Check sheet for the modelled part. Datum: model origin and axes. Units: mm. Give positions to 0.01 mm unless a question says otherwise; leave off trailing zeros. Loops run counter-clockwise (first coordinate to the right, second up) from the corner with the lowest first, then second, coordinate; pieces in that order, holes last.
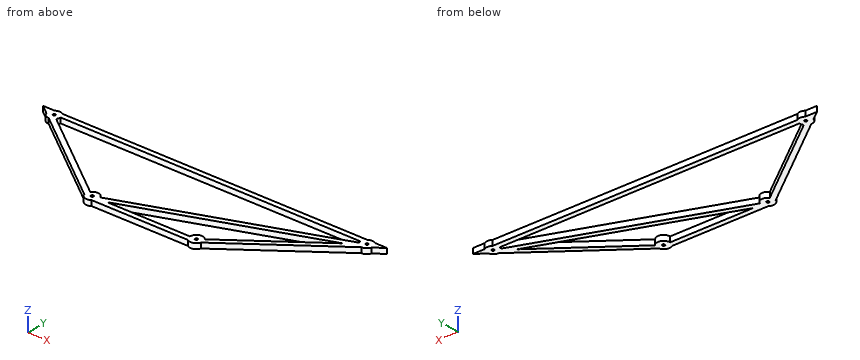
```python
from build123d import *

# Parameters (mm, degrees)
EXTRUDE_THIN2_DEPTH = 20
SKETCH4_R           = 5
CUT_EXTRUDE1_DEPTH  = 1302.393483924


# Read off the part's stored shape, not the designer's step: Extrude-Thin2
with BuildPart() as part:
    # Extrude-Thin2 outline → Extrude-Thin2 (new body)
    with BuildSketch(Plane.XY):
        with BuildLine():
            Line((-15, 20), (-60, 20))
            Line((-60, 20), (-24, -7))
            ThreePointArc((-24, -7), (-15, -20), (0, -25))
            Line((0, -25), (376, -307))
            ThreePointArc((376, -307), (392.09430585, -323.717082451), (415, -320))
            Line((415, -320), (785, -320))
            ThreePointArc((785, -320), (807.90569415, -323.717082451), (824, -307))
            Line((824, -307), (1200, -25))
            ThreePointArc((1200, -25), (1215, -20), (1224, -7))
            Line((1224, -7), (1260, 20))
            Line((1260, 20), (1215, 20))
            ThreePointArc((1215, 20), (1200, 25), (1185, 20))
            Line((1185, 20), (15, 20))
            ThreePointArc((15, 20), (0, 25), (-15, 20))
        make_face()
        with BuildLine():
            Line((456.960024969, -300), (1143.039975031, -42.720018727))
            Line((1143.039975031, -42.720018727), (820, -285))
            ThreePointArc((820, -285), (792.09430585, -276.282917549), (775, -300))
            Line((775, -300), (456.960024969, -300))
        make_face(mode=Mode.SUBTRACT)
        with BuildLine():
            ThreePointArc((1175, 0), (1175.401161247, -4.460620138), (1176.591770561, -8.77808604))
            Line((1176.591770561, -8.77808604), (423.408229439, -291.22191396))
            ThreePointArc((423.408229439, -291.22191396), (403.547120002, -275.252920583), (380, -285))
            Line((380, -285), (20, -15))
            ThreePointArc((20, -15), (23.717082451, -7.90569415), (25, 0))
            Line((25, 0), (1175, 0))
        make_face(mode=Mode.SUBTRACT)
    extrude(amount=EXTRUDE_THIN2_DEPTH)

    # Sketch4 → Cut-Extrude1 (cut, through all)
    with BuildSketch(Plane.XY.offset(20)):
        Circle(SKETCH4_R)
        with Locations((400, -300)):
            Circle(SKETCH4_R)
        with Locations((800, -300)):
            Circle(SKETCH4_R)
        with Locations((1200, 0)):
            Circle(SKETCH4_R)
    extrude(amount=-CUT_EXTRUDE1_DEPTH, mode=Mode.SUBTRACT)


solid = part.part
```
(1) Gauge pin test, flat ends, axial feed: pin 1 Ø2 at (x, z) = (144.5, 11) entering from +Y; pin 2 Ø6 at (x, z) = (515, 11.5) entering from -Y; pin 3 Ø12 at (y, z) = (-17, 12.5) entering from +X. Record the tip position at first contact, or that the pin passes through.
(2) Section check A-A on z = 13. Record the boundary of the cut face in (x, y), plus the area to 3 significant figures.
(3) Material ranges on line 1 (Y direction, x = 400, z = 8.25); line 2 (Y direction, x = 601.5, z = 5.25); line 3 (Y direction, x = 1200, z = 13), recorded low to high.
(4) Section check D-D on x = 654.5. Record the boundary of the cut face in (y, z).
(5) Section check C-C on y = -112.5. Record the boundary of the cut face in (x, z).
(6) Section check B-B on x = 89.5. Record the boundary of the cut face in (y, z) (3 decimals), plus the area to 3 significant figures.
Computed values:
1. pin 1: stops at y = 20
1. pin 2: stops at y = -320
1. pin 3: stops at x = 1222.45
2. outline: (-60, 20) - (-24, -7) arc R25 ccw to (0, -25) - (376, -307) arc R25 ccw to (415, -320) - (785, -320) arc R25 ccw to (824, -307) - (1200, -25) arc R25 ccw to (1224, -7) - (1260, 20) - (1215, 20) arc R25 ccw to (1185, 20) - (15, 20) arc R25 ccw to (-15, 20) - close; hole circle Ø10 at (0, 0); hole (20, -15) - (380, -285) arc R25 cw to (423.41, -291.22) - (1176.59, -8.78) arc R25 cw to (1175, 0) - (25, 0) arc R25 cw to start; hole circle Ø10 at (400, -300); hole (456.96, -300) - (775, -300) arc R25 cw to (820, -285) - (1143.04, -42.72) - close; hole circle Ø10 at (800, -300); hole circle Ø10 at (1200, 0)
2. area: 72,700 mm2
3. line 1: y = -325 to -305, -295 to -275, 0 to 20
3. line 2: y = -320 to -300, -245.8 to -224.44, 0 to 20
3. line 3: y = -25 to -5, 5 to 25
4. outline: (-320, 0) - (-300, 0) - (-300, 20) - (-320, 20) - close; (-225.92, 0) - (-204.56, 0) - (-204.56, 20) - (-225.92, 20) - close; (0, 0) - (20, 0) - (20, 20) - (0, 20) - close
5. outline: (116.67, 0) - (150, 0) - (150, 20) - (116.67, 20) - close; (900, 0) - (956.96, 0) - (956.96, 20) - (900, 20) - close; (1050, 0) - (1083.33, 0) - (1083.33, 20) - (1050, 20) - close
6. outline: (-92.125, 0) - (-67.125, 0) - (-67.125, 20) - (-92.125, 20) - close; (0, 0) - (20, 0) - (20, 20) - (0, 20) - close
6. area: 900 mm2
